from build123d import *

# Parameters (mm, degrees)
CROQUIS1_W              = 20
CROQUIS1_H              = 40
SALIENTE_EXTRUIR1_DEPTH = 8
CROQUIS2_W              = 13
CROQUIS2_H              = 15
CORTAR_EXTRUIR1_DEPTH   = 8
CHAFL_N3_SIZE           = 5
CHAFL_N4_SIZE           = 5
CROQUIS4_W              = 10
CROQUIS4_H              = 8
SALIENTE_EXTRUIR2_DEPTH = 50


with BuildPart() as part:
    # Croquis1 → Saliente-Extruir1 (new body)
    with BuildSketch(Plane.XY):
        Rectangle(CROQUIS1_W, CROQUIS1_H)
    extrude(amount=SALIENTE_EXTRUIR1_DEPTH)

    # Croquis2 → Cortar-Extruir1 (cut)
    with BuildSketch(Plane(origin=(0, 0, 0), x_dir=(-1, 0, 0), z_dir=(0, 0, -1))):
        with Locations((0, 12.5)):
            Rectangle(CROQUIS2_W, CROQUIS2_H)
    extrude(amount=-CORTAR_EXTRUIR1_DEPTH, mode=Mode.SUBTRACT)

    # Chaflán3
    chafl_n3_edges = [part.edges().sort_by_distance(p)[0] for p in [
        (-10, -20, 4),
    ]]
    chamfer(chafl_n3_edges, length=CHAFL_N3_SIZE)

    # Chaflán4
    chafl_n4_edges = [part.edges().sort_by_distance(p)[0] for p in [
        (10, -20, 4),
    ]]
    chamfer(chafl_n4_edges, length=CHAFL_N4_SIZE)

    # Croquis4 → Saliente-Extruir2 (add)
    with BuildSketch(Plane.XZ.offset(20)):
        with Locations((0, 4)):
            Rectangle(CROQUIS4_W, CROQUIS4_H)
    extrude(amount=SALIENTE_EXTRUIR2_DEPTH)


solid = part.part
Model file for the job. Use its own axes, mm. A direction names the side the tool comes from. Give positions to 0.01 mm unless a question says otherwise; leave off trailing zeros. Write each loop counter-clockwise with the first axis right and the second up, starting at its lowest first coordinate (ties: lowest second). Pieces come first, ordered by that corner, then holes. Notation, with made-up numbers: M 4.25,21.25 L 11.25,21.25 A31 ccw 11.25,54.25 Z; hole C 14,-7.5 d2. An arc over 180 degrees is marked long. One line per item, written item: value. Start each with the question number.
Q1. Two-plate mould, pull along X, no slides. Class faces 1 (the flat face through (10, 2, 4)), 2 (the flat face through (-6.5, 12, 4)), 3 (the flat face through (0, -70, 4)): +X half, -X half, draft (parallel to the pull), parting line (faces both ways), or undercut.
Q2. 3-axis set-ups, long thin cutter, end or side, ignore diameter. For faces 4 (the flat face through (5, -45, 4)), 5 (the flat face through (0, 5, 4)), 6 (the flat face through (0, -24, 8)), 7 (the flat face through (-5, -45, 4)): which of +Z, -Z, +X, -X, +Y, -Y reach the whole face in a straight line?
Q3. Drop flat-ended pins along their axis: pin 1 Ø2.5 at (x, z) = (1, 5.5) entering from +Y; pin 2 Ø2.5 at (y, z) = (-48, 5.5) entering from +X; pin 3 Ø4 at (y, z) = (-45.5, 5.5) entering from -X. Give the stop position or say it passes through.
Q4. Saw through at C-C, the plane y = -62.5. Write the cut outline in (x, z).
Q5. Probe probe 1 along X at (y, z) = (10, 5.25); probe 2 along Y at (x, z) = (-1.75, 5.75); probe 3 along X at (y, z) = (-54.5, 6.5). List the from-to ranges inside material, lowest first. Write a range as [from, to].
Q6. Saw through at B-B, the plane x = 7.25. Write the cut outline in (y, z), plus the area to 3 significant figures.
Q7. Saw through at A-A, the plane z = 1.5. Write the cut outline in (x, y), plus the area to 3 significant figures.
Output values:
1. face 1: +X half
1. face 2: undercut
1. face 3: draft
2. face 4: +Z, -Z, +X, -Y
2. face 5: +Z, -Z, +Y
2. face 6: +Z, +X, -X, +Y, -Y
2. face 7: +Z, -Z, -X, -Y
3. pin 1: stops at y = 5
3. pin 2: stops at x = 5
3. pin 3: stops at x = -5
4. outline: M -5,0 L 5,0 L 5,8 L -5,8 Z
5. probe 1: x = [-10, -6.5], [6.5, 10]
5. probe 2: y = [-70, 5]
5. probe 3: x = [-5, 5]
6. outline: M -17.75,0 L 20,0 L 20,8 L -17.75,8 Z
6. area: 302 mm²
7. outline: M -10,-15 L -5,-20 L -5,-70 L 5,-70 L 5,-20 L 10,-15 L 10,20 L 6.5,20 L 6.5,5 L -6.5,5 L -6.5,20 L -10,20 Z
7. area: 1,080 mm²
